Read the model definition and answer for the solid it produces. Units are mm, in the model's axes. A direction names the side the tool comes from. Give positions to 0.01 mm unless a question says otherwise; leave off trailing zeros. Loops run counter-clockwise (first coordinate to the right, second up) from the corner with the lowest first, then second, coordinate; pieces in that order, holes last. Notation, with made-up numbers: (55.5, 15) - (80.5, 15) arc R14 ccw to (80.5, 19) - close; hole circle Ø1 at (8, -31.75). An arc over 180 degrees is marked (long way). Write item = value, one per line.
```python
from build123d import *

# Parameters (mm, degrees)
SKETCH1_W                      = 32.5
SKETCH1_H                      = 80.25
BOSS_EXTRUDE1_DEPTH            = 6
BOSS_EXTRUDE2_DEPTH            = 11
F_6_0MM_DOWEL_HOLE1_D          = 6
M5X0_8_TAPPED_HOLE1_D          = 4.2
CBORE_FOR_M3_SHCS1_D           = 3.4
CBORE_FOR_M3_SHCS1_CBORE_D     = 6.5
CBORE_FOR_M3_SHCS1_CBORE_DEPTH = 3
F_1_0_1_DIAMETER_HOLE1_D       = 1
SKETCH12_R                     = 1.5
CUT_EXTRUDE1_DEPTH             = 5
SKETCH13_W                     = 6
SKETCH13_H                     = 35
CUT_EXTRUDE2_DEPTH             = 69.184034055
FILLET1_R                      = 2.38125
SKETCH14_W                     = 34.5
SKETCH14_H                     = 82.25
CUT_EXTRUDE3_DEPTH             = 69.184034055
M3X0_5_START                   = -6
M3X0_5_TAPPED_HOLE1_OUTLINE_R  = 1.25
M3X0_5_TAPPED_HOLE1_DEPTH      = 17


# Read off the part's stored shape, not the designer's step: M3x0.5 Tapped Hole1
with BuildPart() as part:
    # Sketch1 → Boss-Extrude1 (new body)
    with BuildSketch(Plane(origin=(0, 0, 0), x_dir=(1, 0, 0), z_dir=(0, 1, 0))):
        with Locations((0, -23.875)):
            Rectangle(SKETCH1_W, SKETCH1_H)
    extrude(amount=-BOSS_EXTRUDE1_DEPTH)

    # Sketch2 → Boss-Extrude2 (add)
    with BuildSketch(Plane(origin=(0, 0, 0), x_dir=(1, 0, 0), z_dir=(0, 1, 0))):
        with BuildLine():
            Line((-5.032198748, 16.25), (5.032198748, 16.25))
            ThreePointArc((5.032198748, 16.25), (1.230950737, -7.608861929), (16.25, -26.532998323))
            Line((16.25, -26.532998323), (16.25, -64))
            Line((16.25, -64), (-16.25, -64))
            Line((-16.25, -64), (-16.25, -26.532998323))
            ThreePointArc((-16.25, -26.532998323), (-1.230950737, -7.608861929), (-5.032198748, 16.25))
        make_face()
    extrude(amount=BOSS_EXTRUDE2_DEPTH)

    # Ø6.0mm Dowel Hole1 (through all)
    with Locations(Plane(origin=(16.25, 0, 0), x_dir=(0, 0, -1), z_dir=(1, 0, 0))):
        with Locations((-57, 6), (-39, 6)):
            Hole(F_6_0MM_DOWEL_HOLE1_D / 2)

    # M5x0.8 Tapped Hole1 (through all)
    with Locations(Plane(origin=(16.25, 0, 0), x_dir=(0, 0, -1), z_dir=(1, 0, 0))):
        with Locations((-48, 6)):
            Hole(M5X0_8_TAPPED_HOLE1_D / 2)

    # CBORE for M3 SHCS1 (through all)
    with Locations(Plane(origin=(0, 0, 0), x_dir=(1, 0, 0), z_dir=(0, 1, 0))):
        with Locations((-11, 11), (11, 11), (11, -11), (-11, -11)):
            CounterBoreHole(CBORE_FOR_M3_SHCS1_D / 2, CBORE_FOR_M3_SHCS1_CBORE_D / 2, CBORE_FOR_M3_SHCS1_CBORE_DEPTH)

    # Ø1.0 (1) Diameter Hole1 (through all)
    with Locations(Plane(origin=(0, 11, 0), x_dir=(1, 0, 0), z_dir=(0, 1, 0))):
        with Locations((0, 0)):
            Hole(F_1_0_1_DIAMETER_HOLE1_D / 2)

    # Sketch12 → Cut-Extrude1 (cut)
    with BuildSketch(Plane.XZ.offset(6)):
        with Locations(Location((0, 0, 0), (0, 0, 270))):
            Circle(SKETCH12_R)
    extrude(amount=-CUT_EXTRUDE1_DEPTH, mode=Mode.SUBTRACT)

    # Sketch13 → Cut-Extrude2 (cut, through all)
    with BuildSketch(Plane(origin=(0, 11, 0), x_dir=(1, 0, 0), z_dir=(0, 1, 0))):
        with Locations((-13.25, -46.5)):
            Rectangle(SKETCH13_W, SKETCH13_H)
        with Locations((13.25, -46.5)):
            Rectangle(SKETCH13_W, SKETCH13_H)
    extrude(amount=-CUT_EXTRUDE2_DEPTH, mode=Mode.SUBTRACT)

    # Fillet1
    fillet1_edges = [part.edges().sort_by_distance(p)[0] for p in [
        (-10.25, 2.5, 29),
        (10.25, 2.5, 29),
    ]]
    fillet(fillet1_edges, radius=FILLET1_R)

    # Sketch14 → Cut-Extrude3 (cut, through all)
    with BuildSketch(Plane(origin=(0, 11, 0), x_dir=(1, 0, 0), z_dir=(0, 1, 0))):
        with Locations((0, -23.875)):
            Rectangle(SKETCH14_W, SKETCH14_H)
        with BuildLine():
            Line((-7.5, -63.5), (-7.5, -19.94427191))
            ThreePointArc((-7.5, -19.94427191), (-8.645898034, -16.94427191), (-11.5, -15.472135955))
            ThreePointArc((-11.5, -15.472135955), (-14.354101966, -14), (-15.5, -11))
            Line((-15.5, -11), (-15.5, 11))
            ThreePointArc((-15.5, 11), (-14.181980515, 14.181980515), (-11, 15.5))
            Line((-11, 15.5), (11, 15.5))
            ThreePointArc((11, 15.5), (14.181980515, 14.181980515), (15.5, 11))
            Line((15.5, 11), (15.5, -11))
            ThreePointArc((15.5, -11), (14.354101966, -14), (11.5, -15.472135955))
            ThreePointArc((11.5, -15.472135955), (8.645898034, -16.94427191), (7.5, -19.94427191))
            Line((7.5, -19.94427191), (7.5, -63.5))
            Line((7.5, -63.5), (-7.5, -63.5))
        make_face(mode=Mode.SUBTRACT)
    extrude(amount=-CUT_EXTRUDE3_DEPTH, mode=Mode.SUBTRACT)

    # M3x0.5 Tapped Hole1 outline → M3x0.5 Tapped Hole1 (cut)
    with BuildSketch(Plane(origin=(0, 0, 0), x_dir=(1, 0, 0), z_dir=(0, 1, 0)).offset(M3X0_5_START)):
        with Locations((0, -12.5)):
            Circle(M3X0_5_TAPPED_HOLE1_OUTLINE_R)
        with Locations((0, 12.5)):
            Circle(M3X0_5_TAPPED_HOLE1_OUTLINE_R)
    extrude(amount=M3X0_5_TAPPED_HOLE1_DEPTH, mode=Mode.SUBTRACT)


solid = part.part
```
1) Each of these flat-tipped pins is pushed along its axis until it touches: P1, Ø3, axis at x = -11, z = -11, coming from the +Y side; P2, Ø3, axis at x = -11.5, z = 12.5, coming from the +Y side; P3, Ø2, axis at y = 2.5, z = -1.5, coming from the +X side; P4, Ø4.5, axis at x = -7, z = 2.5, coming from the +Y side. Where does it stop, or does it pass through?
Output:
P1 = through
P2 = -3
P3 = 0.35
P4 = 0
2) A cutting plane is placed at C-C on z = 39. Determine the outline of the cut face in (x, y).
Output:
outline = (-7.5, -6) - (7.5, -6) - (7.5, 3) - (-7.5, 3) - close; (-7.5, 9) - (7.5, 9) - (7.5, 11) - (-7.5, 11) - close
3) The mould has two halves that part along Y. Classify faces 5 (the face through (0, 6, 54)), 6 (the face through (10.2, -4.5, 12.5)), 7 (the face through (12.4, -3, -9.6)): pulls with the +Y half, pulls with the -Y half, needs draft (parallel to the pull), parting line crosses it, or undercut.
Output:
face_5 = undercut
face_6 = needs draft
face_7 = pulls with the +Y half
4) Find the intervals of material crossed by probe 1 along Z at (x, y) = (0, 2.5); probe 2 along Z at (x, y) = (3, 8.5); probe 3 along X at (y, z) = (-1.25, -8), in increasing order.
Output:
probe_1 = -15.5 to -13.75, -11.25 to -0.5, 0.5 to 11.25, 13.75 to 63.5
probe_2 = -15.5 to -12.55, 12.55 to 37.34, 40.66 to 55.34, 58.66 to 63.5
probe_3 = -15.5 to -12.25, -9.75 to 9.75, 12.25 to 15.5
5) A cutting plane is placed at D-D on y = -2. Determine the outline of the cut face in (x, z), then the cut area to 3 significant figures.
Output:
outline = (-15.5, -11) arc R4.5 ccw to (-11, -15.5) - (11, -15.5) arc R4.5 ccw to (15.5, -11) - (15.5, 11) arc R4.5 ccw to (11.5, 15.47) arc R4.5 cw to (7.5, 19.94) - (7.5, 63.5) - (-7.5, 63.5) - (-7.5, 19.94) arc R4.5 cw to (-11.5, 15.47) arc R4.5 ccw to (-15.5, 11) - close; hole circle Ø6.5 at (-11, -11); hole circle Ø6.5 at (-11, 11); hole circle Ø3 at (0, 0); hole circle Ø2.5 at (0, -12.5); hole circle Ø2.5 at (0, 12.5); hole circle Ø6.5 at (11, -11); hole circle Ø6.5 at (11, 11)
area = 1,520 mm²
6) A cutting plane is placed at B-B on y = 6. Determine the outline of the cut face in (x, z), then the cut area to 3 significant figures.
Output:
outline = (-7.52, 19.57) arc R30 cw to (-0.25, 0.43) arc R0.5 cw to (0.25, 0.43) arc R30 cw to (7.52, 19.57) arc R4.5 cw to (7.5, 19.94) - (7.5, 36) - (-7.5, 36) - (-7.5, 19.94) arc R4.5 cw to start; (-7.5, 42) - (7.5, 42) - (7.5, 45.9) - (-7.5, 45.9) - close; (-7.5, 50.1) - (7.5, 50.1) - (7.5, 54) - (-7.5, 54) - close; (-7.5, 60) - (7.5, 60) - (7.5, 63.5) - (-7.5, 63.5) - close; (-4.56, -15.5) - (4.56, -15.5) arc R30 cw to (0.25, -0.43) arc R0.5 cw to (-0.25, -0.43) arc R30 cw to start; hole circle Ø2.5 at (0, -12.5); hole circle Ø2.5 at (0, 12.5)
area = 556 mm²
7) A tool of negligible diameter and unlimited length cuts with its end or side. For faces 1 (the face through (-7.5, 3, 42)), 2 (the face through (7.5, 3, 41)), 3 (the face through (2.149, 5.423, 10.504)), 4 (the face through (-8, 0, 2)), from which of +Z, -Z, +X, -X, +Y, -Y can it reach the whole face along a straight path? Write none if from no direction.
Output:
face_1 = +Z, -X, +Y, -Y
face_2 = +Z, +X, +Y, -Y
face_3 = +X, +Y
face_4 = -X, +Y
8) A cutting plane is placed at A-A on z = 48. Determine the outline of the cut face in (x, y).
Output:
outline = (-7.5, -6) - (7.5, -6) - (7.5, 3.9) - (-7.5, 3.9) - close; (-7.5, 8.1) - (7.5, 8.1) - (7.5, 11) - (-7.5, 11) - close
